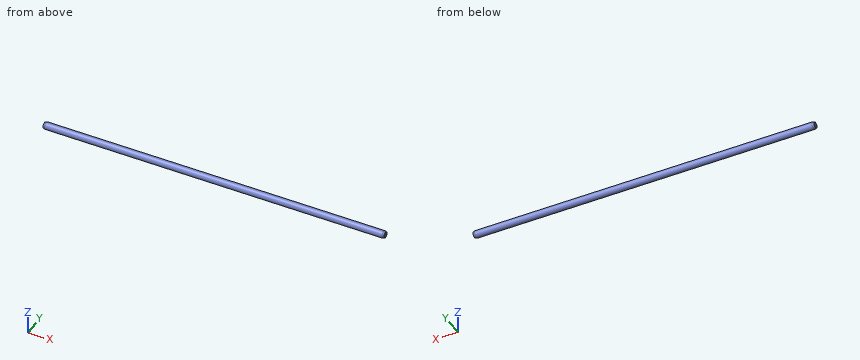
```python
from build123d import *

# Parameters (mm, degrees)
SKETCH1_R           = 4
BOSS_EXTRUDE1_DEPTH = 194.5
CHAMFER3_SIZE       = 2
CHAMFER3_SIZE2      = 0.535898385
CHAMFER4_SIZE       = 2
CHAMFER4_SIZE2      = 0.535898385


with BuildPart() as part:
    # Sketch1 → Boss-Extrude1 (new body, symmetric)
    with BuildSketch(Plane(origin=(0, 0, 0), x_dir=(0, 0, -1), z_dir=(1, 0, 0))):
        Circle(SKETCH1_R)
    extrude(amount=BOSS_EXTRUDE1_DEPTH, both=True)

    # Chamfer3
    chamfer3_edges = [part.edges().sort_by_distance(p)[0] for p in [
        (194.5, 0, 4),
    ]]
    chamfer3_side = [part.faces().sort_by_distance(p)[0] for p in [
        (0, 0, 4),
    ]]
    chamfer(chamfer3_edges, length=CHAMFER3_SIZE, length2=CHAMFER3_SIZE2, reference=chamfer3_side[0])

    # Chamfer4
    chamfer4_edges = [part.edges().sort_by_distance(p)[0] for p in [
        (-194.5, 0, 4),
    ]]
    chamfer4_side = [part.faces().sort_by_distance(p)[0] for p in [
        (-1, 0, 4),
    ]]
    chamfer(chamfer4_edges, length=CHAMFER4_SIZE, length2=CHAMFER4_SIZE2, reference=chamfer4_side[0])


solid = part.part
```
Design review of the part built by this model. Coordinates are the model's own, in mm. Round coordinates to 2 decimals unless told otherwise and drop trailing zeros. Write each loop counter-clockwise with the first axis right and the second up, starting at its lowest first coordinate (ties: lowest second). Pieces come first, ordered by that corner, then holes.
Item 1: For probe 1 along Z at (x, y) = (66, 2); probe 2 along Y at (x, z) = (-131, -1.5); probe 3 along Y at (x, z) = (152, 0.5), list the stretches that pass through material, from the lowest coordinate up.
Item 2: We need section A-A on x = 51. Write out the cut boundary in (y, z), and give its area (3 significant figures).
Item 3: Clearance check with a flat-ended pin moving along its axis: pin 1 Ø3 at (x, z) = (70, 2.5) entering from -Y. State where the tip first meets the part, or that it passes through.
Returned:
1. probe 1: z = -3.46 to 3.46
1. probe 2: y = -3.71 to 3.71
1. probe 3: y = -3.97 to 3.97
2. outline: circle Ø8 at (0, 0)
2. area: 50.3 mm2
3. pin 1: stops at y = -3.87
